from build123d import *

# Parameters (mm, degrees)
SKETCH1_R           = 0.375
BOSS_EXTRUDE1_DEPTH = 0.1


with BuildPart() as part:
    # Sketch1 → Boss-Extrude1 (new body, symmetric)
    with BuildSketch(Plane.XY):
        with BuildLine():
            Line((-4, 8.75), (-0.829156198, 8.75))
            ThreePointArc((-0.829156198, 8.75), (0, 11.5), (0.829156198, 8.75))
            Line((0.829156198, 8.75), (4, 8.75))
            Line((4, 8.75), (4, 8.25))
            Line((4, 8.25), (1.070800598, 1.663056339))
            ThreePointArc((1.070800598, 1.663056339), (3.990187346, -3.645423064), (0.468669321, -8.575096822))
            ThreePointArc((0.468669321, -8.575096822), (0.367162541, -11.454369853), (-1.088850392, -8.968300032))
            ThreePointArc((-1.088850392, -8.968300032), (-2.57467118, -8.930560768), (-4, -8.509223116))
            Line((-4, -8.509223116), (-3.796834113, -8.052360311))
            ThreePointArc((-3.796834113, -8.052360311), (3.052360311, -5.419717925), (0.419717925, 1.429476498))
            Line((0.419717925, 1.429476498), (3.452789771, 8.25))
            Line((3.452789771, 8.25), (-4, 8.25))
            Line((-4, 8.25), (-4, 8.75))
        make_face()
        with Locations((0, 10)):
            Circle(SKETCH1_R, mode=Mode.SUBTRACT)
        with Locations((0, -10)):
            Circle(SKETCH1_R, mode=Mode.SUBTRACT)
    extrude(amount=BOSS_EXTRUDE1_DEPTH, both=True)


solid = part.part
CAD build for the part. Positions are in the model's coordinates, mm. Coordinates: 2 decimals unless noted, no trailing zeros. Loops run counter-clockwise (first coordinate to the right, second up) from the corner with the lowest first, then second, coordinate; pieces in that order, holes last. Notation, with made-up numbers: (51, 67.5) - (60, 67.5) arc R29 ccw to (60, 98.5) - close; hole circle Ø2 at (74, 80.5). An arc over 180 degrees is marked (long way). Write item = value, one per line. Start each with the question number.
Q1. Cut at D-D, the plane x = 2. List the corners of the cut face in (y, z), then the cut area to 3 significant figures.
Q2. Cut at B-B, the plane x = 0. List the corners of the cut face in (y, z) (3 decimals).
Q3. Cut at A-A, the plane y = -10. List the corners of the cut face in (x, z) (3 decimals).
Q4. Drill centre lines: L1, parallel to Y at x = 0, z = 0 (3 decimals); L2, parallel to Y at x = 0.75, z = 0; L3, parallel to Y at x = -0.5, z = 0. Where is each one in solid material? Low to high.
Computed:
q1.outline = (-7.64, -0.1) - (-6.96, -0.1) - (-6.96, 0.1) - (-7.64, 0.1) - close; (0.34, -0.1) - (1.02, -0.1) - (1.02, 0.1) - (0.34, 0.1) - close; (3.75, -0.1) - (4.98, -0.1) - (4.98, 0.1) - (3.75, 0.1) - close; (8.25, -0.1) - (8.75, -0.1) - (8.75, 0.1) - (8.25, 0.1) - close
q1.area = 0.619 mm²
q2.outline = (-11.5, -0.1) - (-10.375, -0.1) - (-10.375, 0.1) - (-11.5, 0.1) - close; (-9.625, -0.1) - (-8.218, -0.1) - (-8.218, 0.1) - (-9.625, 0.1) - close; (8.25, -0.1) - (9.625, -0.1) - (9.625, 0.1) - (8.25, 0.1) - close; (10.375, -0.1) - (11.5, -0.1) - (11.5, 0.1) - (10.375, 0.1) - close
q3.outline = (-1.5, -0.1) - (-0.375, -0.1) - (-0.375, 0.1) - (-1.5, 0.1) - close; (0.375, -0.1) - (1.5, -0.1) - (1.5, 0.1) - (0.375, 0.1) - close
q4.L1 = -11.5 to -10.375, -9.625 to -8.218, 8.25 to 9.625, 10.375 to 11.5
q4.L2 = -11.3 to -8.7, -8.45 to -7.89, 1.27 to 2.17, 8.25 to 11.3
q4.L3 = -11.41 to -8.36, 8.25 to 11.41
